Design review of the part shown in the three views and the two pictorial views. Dimensions are in mm from the part's minimum x, y and z. A direction names the side the tool comes from. Give positions to 0.01 mm unless a question says otherwise; leave off trailing zeros. Order: outer loops, then holes, each group sorted by start corner. A loop starts at its lowest first (then second) coordinate and runs counter-clockwise, first axis right, second up.
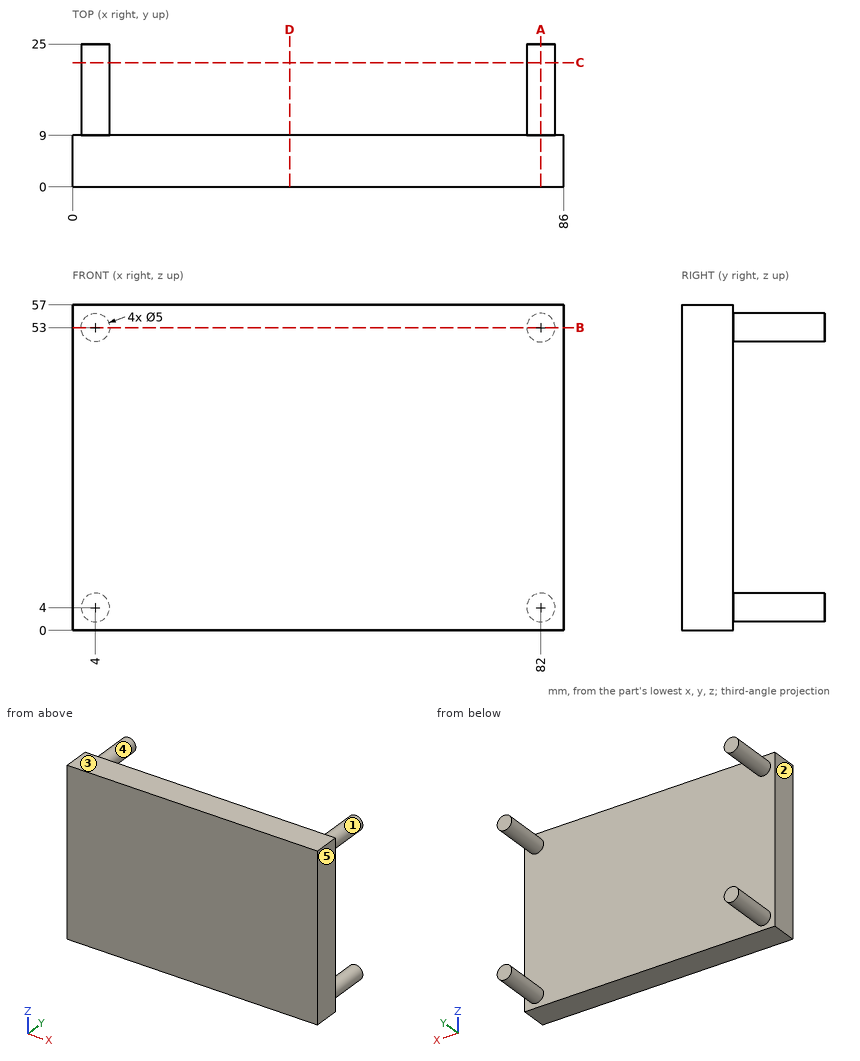
1) Clearance check with flat-ended pins moving along their axes: pin 1 (3 mm diameter, centred on x = 62, y = 12, fed in from -Z); pin 2 (3 mm diameter, centred on x = 69.5, z = 32, fed in from +Y). State where each tip first meets the part, or that it passes through.
Answer sheet:
pin 1: passes through
pin 2: stops at y = 9
2) Tool access review of the marked faces 4 and 5: name each direction out of +Z, -Z, +X, -X, +Y, -Y from which nothing blocks a thin tool from reaching the whole face with its end or side.
Answer sheet:
face 4: +Y
face 5: +Z, -Z, +X, +Y, -Y
3) We need section C-C on y = 21.75. Give the boundary of the cut face in (x, z), then the cut area to 3 significant figures.
Answer sheet:
outline: circle Ø5 at (4, 4); circle Ø5 at (4, 53); circle Ø5 at (82, 4); circle Ø5 at (82, 53)
area: 78.5 mm2
4) We need section B-B on z = 53. Give the boundary of the cut face in (x, y).
Answer sheet:
outline: (0, 0) - (86, 0) - (86, 9) - (84.5, 9) - (84.5, 25) - (79.5, 25) - (79.5, 9) - (6.5, 9) - (6.5, 25) - (1.5, 25) - (1.5, 9) - (0, 9) - close
5) To check wall thickness, follow line 1 (Y direction, x = 36.5, z = 40.5); line 2 (X direction, y = 19, z = 52); line 3 (X direction, y = 18.25, z = 6). State the ranges of each line that lie inside material, in increasing order.
Answer sheet:
line 1: y = 0 to 9
line 2: x = 1.71 to 6.29, 79.71 to 84.29
line 3: x = 2.5 to 5.5, 80.5 to 83.5
6) We need section D-D on x = 38. Give the boundary of the cut face in (y, z), then the cut area to 3 significant figures.
Answer sheet:
outline: (0, 0) - (9, 0) - (9, 57) - (0, 57) - close
area: 513 mm2
7) We need section A-A on x = 82. Give the boundary of the cut face in (y, z), then the cut area to 3 significant figures.
Answer sheet:
outline: (0, 0) - (9, 0) - (9, 1.5) - (25, 1.5) - (25, 6.5) - (9, 6.5) - (9, 50.5) - (25, 50.5) - (25, 55.5) - (9, 55.5) - (9, 57) - (0, 57) - close
area: 673 mm2
8) Draft analysis for pull direction Z (two halves, no side actions). For the marked faces 1, 2 and 3, state which applies: +Z half, -Z half, draft (parallel to the pull), parting line (faces both ways), or undercut.
Answer sheet:
face 1: undercut
face 2: draft
face 3: +Z half
